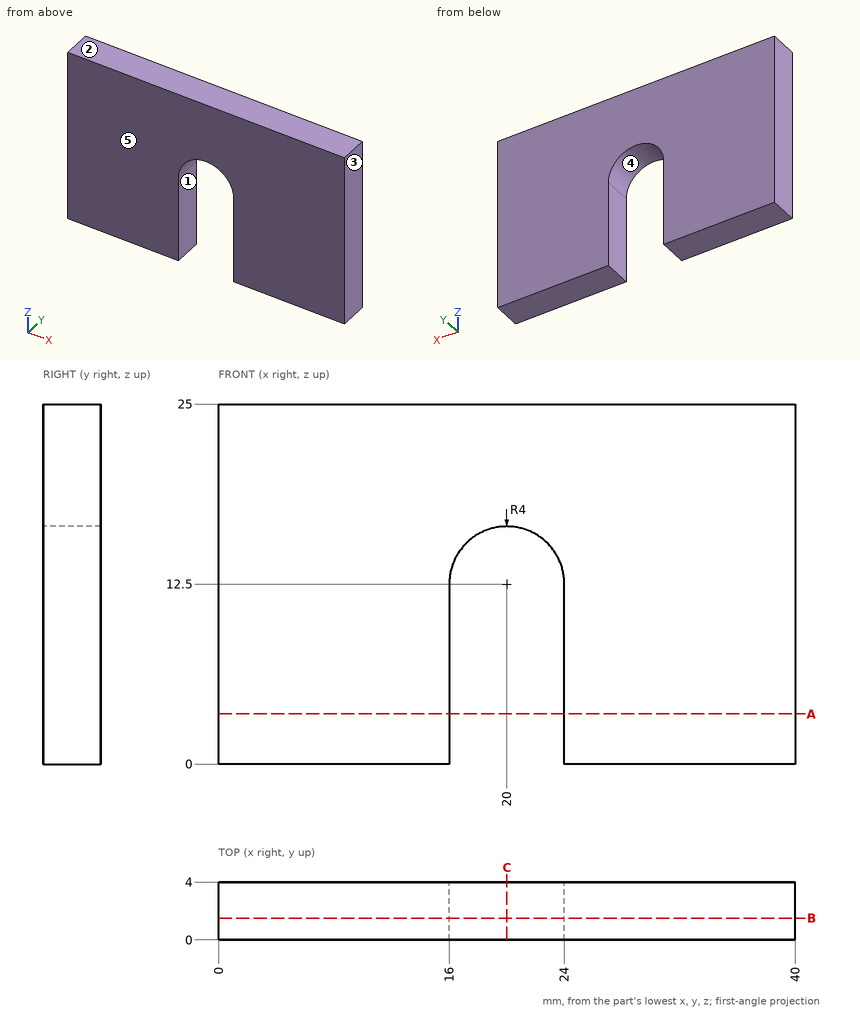
Check sheet for the drawn part. Datum: minimum x, y, z corner. Units: mm. A direction names the side the tool comes from. Give positions to 0.01 mm unless a question says otherwise; leave off trailing zeros. Loops run counter-clockwise (first coordinate to the right, second up) from the corner with the lowest first, then second, coordinate; pieces in that order, holes last.
1) Draft check along X on the marked faces 3, 4 and 5. Enter one of: pulls with the +X half, pulls with the -X half, needs draft (parallel to the pull), parting line crosses it, or undercut.
2) Sectioned sample at C-C, the plane x = 20. Enter the section's corners in (y, z).
3) Thickness scan on line 1 along X through (y, z) = (3.15, 2.75); line 2 along X through (y, z) = (0.75, 14); line 3 along Z through (x, y) = (22, 2.95). Record the ranges inside material, lowest first.
4) Sectioned sample at A-A, the plane z = 3.5. Enter the section's corners in (x, y), then the cut area to 3 significant figures.
5) Sectioned sample at B-B, the plane y = 1.5. Enter the section's corners in (x, z), then the cut area to 3 significant figures.
6) Set-up check for the marked faces 1 and 2: record each of +Z, -Z, +X, -X, +Y, -Y from which the full face is reachable in a straight line by a thin tool's end or side.
Answers:
1. face 3: pulls with the +X half
1. face 4: undercut
1. face 5: needs draft
2. outline: (0, 16.5) - (4, 16.5) - (4, 25) - (0, 25) - close
3. line 1: x = 0 to 16, 24 to 40
3. line 2: x = 0 to 16.29, 23.71 to 40
3. line 3: z = 15.96 to 25
4. outline: (0, 0) - (16, 0) - (16, 4) - (0, 4) - close; (24, 0) - (40, 0) - (40, 4) - (24, 4) - close
4. area: 128 mm2
5. outline: (0, 0) - (16, 0) - (16, 12.5) arc R4 cw to (24, 12.5) - (24, 0) - (40, 0) - (40, 25) - (0, 25) - close
5. area: 875 mm2
6. face 1: -Z, +Y, -Y
6. face 2: +Z, +X, -X, +Y, -Y
